Read the model definition and answer for the solid it produces. Units are mm, in the model's axes. A direction names the side the tool comes from. Give positions to 0.01 mm unless a question says otherwise; leave off trailing zeros. Write each loop counter-clockwise with the first axis right and the second up, starting at its lowest first coordinate (ties: lowest second). Pieces come first, ordered by that corner, then holes. Notation, with made-up numbers: M -11.75,57 L 46.25,57 A11 cw 46.25,68 Z; hole C -36,-5 d6. An arc over 180 degrees is marked long. Put each result on its own line as item: value.
from build123d import *

# Parameters (mm, degrees)
SKETCH1_R           = 1.4
BOSS_EXTRUDE1_DEPTH = 4
CUT_EXTRUDE1_DEPTH  = 9


with BuildPart() as part:
    # Sketch1 → Boss-Extrude1 (new body)
    with BuildSketch(Plane.XY):
        with BuildLine():
            Line((-5, 11.5), (-5, -13.4))
            ThreePointArc((-5, -13.4), (-4.414213562, -14.814213562), (-3, -15.4))
            Line((-3, -15.4), (1, -15.4))
            ThreePointArc((1, -15.4), (2.414213562, -14.814213562), (3, -13.4))
            Line((3, -13.4), (3, 11.5))
            ThreePointArc((3, 11.5), (2.414213562, 12.914213562), (1, 13.5))
            Line((1, 13.5), (-3, 13.5))
            ThreePointArc((-3, 13.5), (-4.414213562, 12.914213562), (-5, 11.5))
        make_face()
        with Locations((0, 10.5)):
            Circle(SKETCH1_R, mode=Mode.SUBTRACT)
        with BuildLine():
            Line((0.964249247, -11.514999207), (-1.035750753, -13.414999207))
            ThreePointArc((-1.035750753, -13.414999207), (-3.014999207, -13.364249247), (-2.964249247, -11.385000793))
            Line((-2.964249247, -11.385000793), (-0.964249247, -9.485000793))
            ThreePointArc((-0.964249247, -9.485000793), (1.014999207, -9.535750753), (0.964249247, -11.514999207))
        make_face(mode=Mode.SUBTRACT)
    extrude(amount=BOSS_EXTRUDE1_DEPTH)

    # Sketch2 → Cut-Extrude1 (cut, through all)
    with BuildSketch(Plane(origin=(3, 0, 0), x_dir=(0, 0, -1), z_dir=(1, 0, 0))):
        Polygon((-4, 6.5), (-2.7, 6.5), (-2.7, 4.5), (-1.5, 4.5), (-1.5, -4.5), (-2.7, -4.5), (-2.7, -6.5), (-4, -6.5), align=None)
    extrude(amount=-CUT_EXTRUDE1_DEPTH, mode=Mode.SUBTRACT)


solid = part.part
(1) Section B-B on y = 10.5 is taken. Determine the outline of the cut face in (x, z).
Result:
outline: M -5,0 L -1.4,0 L -1.4,4 L -5,4 Z; M 1.4,0 L 3,0 L 3,4 L 1.4,4 Z
(2) Which of the six approach directions +Z, -Z, +X, -X, +Y, -Y give full straight-line access (tool end or side, diameter ignored) to faces 4 (the face through (-0.02, -12.45, 1.97)), 5 (the face through (-1, 0, 1.5)), 6 (the face through (-4.4, 12.93, 1.97))?
Result:
face 4: +Z, -Z
face 5: +Z, +X, -X
face 6: +Z, -Z, -X, +Y
(3) Section A-A on z = 3.6 is taken. Determine the outline of the cut face in (x, y) (3 decimals).
Result:
outline: M -5,-13.4 A2 ccw -3,-15.4 L 1,-15.4 A2 ccw 3,-13.4 L 3,-6.5 L -5,-6.5 Z; M -5,6.5 L 3,6.5 L 3,11.5 A2 ccw 1,13.5 L -3,13.5 A2 ccw -5,11.5 Z; hole M -2.964,-11.385 A1.4 ccw -1.036,-13.415 L 0.964,-11.515 A1.4 ccw -0.964,-9.485 Z; hole C 0,10.5 d2.8
(4) Section C-C on x = -2 is taken. Determine the outline of the cut face in (y, z), and give its area (3 significant figures).
Result:
outline: M -15.4,0 L -13.8,0 L -13.8,4 L -15.4,4 Z; M -10.47,0 L 13.5,0 L 13.5,4 L 6.5,4 L 6.5,2.7 L 4.5,2.7 L 4.5,1.5 L -4.5,1.5 L -4.5,2.7 L -6.5,2.7 L -6.5,4 L -10.47,4 Z
area: 74.6 mm²
(5) Straight lines are drawn through the part: line 1 along Y through (x, z) = (-2.75, 2.85); line 2 along Z through (x, y) = (1.75, 2); line 3 along Y through (x, z) = (0, 2.75). For each, find the intervals that lie inside material, in ascending order. Write a range as from..to.
Result:
line 1: y = -15.4..-13.58, -11.18..-6.5, 6.5..13.5
line 2: z = 0..1.5
line 3: y = -15.4..-12.43, -9.1..-6.5, 6.5..9.1, 11.9..13.5
(6) Given pin 1 Ø1 at (x, y) = (-1, 5.5) entering from +Z, flat-ended and moving along its own axis, determine where the tip first touches the part or whether it passes through.
Result:
pin 1: stops at z = 2.7
(7) For a pull along Y with two mould halves and no side action, classify faces 1 (the face through (-1, 6.5, 3)), 2 (the face through (-1, -15.4, 2)), 3 (the face through (-1, 13.5, 2)) as +Y half, -Y half, draft (parallel to the pull), parting line (faces both ways), or undercut.
Result:
face 1: undercut
face 2: -Y half
face 3: +Y half
(8) Section D-D on z = 1.1 is taken. Determine the outline of the cut face in (x, y) (3 decimals).
Result:
outline: M -5,-13.4 A2 ccw -3,-15.4 L 1,-15.4 A2 ccw 3,-13.4 L 3,11.5 A2 ccw 1,13.5 L -3,13.5 A2 ccw -5,11.5 Z; hole M -2.964,-11.385 A1.4 ccw -1.036,-13.415 L 0.964,-11.515 A1.4 ccw -0.964,-9.485 Z; hole C 0,10.5 d2.8
